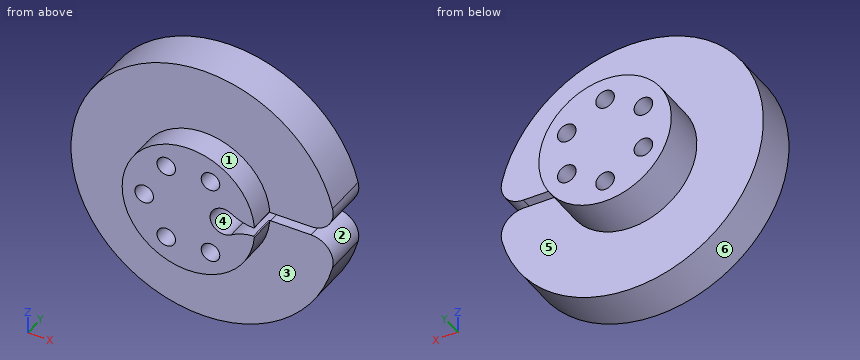
from build123d import *

# Parameters (mm, degrees)
SKETCH_1_R          = 30
EXTRUDE_1_DEPTH     = 10
SKETCH_2_R          = 14.975
EXTRUDE_2_DEPTH     = 10
EXTRUDE_START       = 6
SKETCH_3_R          = 14.975
EXTRUDE_3_DEPTH     = 6
SKETCH_4_R          = 2.1
CUT_EXTRUDE_1_DEPTH = 16
CUT_EXTRUDE_3_DEPTH = 46.343136195
FILLET_1_R          = 10
FILLET_2_R          = 5
FILLET_3_R          = 0.2
SKETCH_7_R          = 1.25
CUT_EXTRUDE_4_DEPTH = 8
SKETCH_8_R          = 2.1
CUT_EXTRUDE_5_DEPTH = 5


with BuildPart() as part:
    # 草图1 → 凸台-拉伸1 (new body)
    with BuildSketch(Plane(origin=(0, 0, 0), x_dir=(1, 0, 0), z_dir=(0, 1, 0))):
        with Locations(Location((0, 0, 0), (0, 0, 270))):
            Circle(SKETCH_1_R)
    extrude(amount=EXTRUDE_1_DEPTH)

    # 草图2 → 凸台-拉伸2 (add)
    with BuildSketch(Plane(origin=(0, 10, 0), x_dir=(1, 0, 0), z_dir=(0, 1, 0))):
        with Locations(Location((0, 0, 0), (0, 0, 270))):
            Circle(SKETCH_2_R)
    extrude(amount=EXTRUDE_2_DEPTH)

    # 草图3 → 凸台-拉伸3 (add)
    with BuildSketch(Plane.XZ.offset(EXTRUDE_START)):
        with Locations(Location((0, 0, 0), (0, 0, 90))):
            Circle(SKETCH_3_R)
    extrude(amount=-EXTRUDE_3_DEPTH)

    # 草图4 → 切除-拉伸1 (cut)
    with BuildSketch(Plane.XZ.offset(6)):
        with Locations(Location((-10, 0, 0), (0, 0, 270))):
            Circle(SKETCH_4_R)
        with Locations(Location((-5, 8.660254038, 0), (0, 0, 270))):
            Circle(SKETCH_4_R)
        with Locations(Location((5, 8.660254038, 0), (0, 0, 270))):
            Circle(SKETCH_4_R)
        with Locations(Location((5, -8.660254038, 0), (0, 0, 270))):
            Circle(SKETCH_4_R)
        with Locations(Location((-5, -8.660254038, 0), (0, 0, 270))):
            Circle(SKETCH_4_R)
    extrude(amount=-CUT_EXTRUDE_1_DEPTH, mode=Mode.SUBTRACT)

    # 草图6 → 切除-拉伸3 (cut, through all)
    with BuildSketch(Plane(origin=(0, 10, 0), x_dir=(1, 0, 0), z_dir=(0, 1, 0))):
        with BuildLine():
            Line((10.93428015, 1), (30.93428015, 1))
            Line((30.93428015, 1), (30.93428015, -1))
            Line((30.93428015, -1), (10.93428015, -1))
            ThreePointArc((10.93428015, -1), (4.9, 0), (10.93428015, 1))
        make_face()
    extrude(amount=-CUT_EXTRUDE_3_DEPTH, mode=Mode.SUBTRACT)

    # 圆角1
    # the kernel refuses this fillet: 10 mm, written as the material it takes off along each edge
    with BuildSketch(Plane(origin=(10.93428015, 10, -1), x_dir=(1, 0, 0), z_dir=(0, -1, 0))) as fillet_1_piece_1:
        with BuildLine():
            CenterArc((4.179790415, -10), FILLET_1_R, 90, 32.892109865)
            ThreePointArc((-1.250797803, -1.603053435), (-0.490230703, -0.906992999), (0, 0))
            Line((0, 0), (4.179790415, 0))
        make_face()
    extrude(amount=26.449476036, mode=Mode.SUBTRACT)
    with BuildSketch(Plane(origin=(10.93428015, 10, 1), x_dir=(1, 0, 0), z_dir=(0, -1, 0))) as fillet_1_piece_2:
        with BuildLine():
            CenterArc((4.179790415, 10), FILLET_1_R, 237.107890135, 32.892109865)
            ThreePointArc((-1.250797803, 1.603053435), (-0.490230703, 0.906992999), (0, 0))
            Line((0, 0), (4.179790415, 0))
        make_face()
    extrude(amount=26.449476036, mode=Mode.SUBTRACT)

    # 圆角2
    fillet_2_edges = [part.edges().sort_by_distance(p)[0] for p in [
        (29.983328701, 5, -1),
        (29.983328701, 5, 1),
    ]]
    fillet(fillet_2_edges, radius=FILLET_2_R)

    # 圆角3
    fillet_3_edges = [part.edges().sort_by_distance(p)[0] for p in [
        (14.941473943, -3, 1.001489591),
        (14.941473943, -3, -1.001489591),
    ]]
    fillet(fillet_3_edges, radius=FILLET_3_R)

    # 草图7 → 切除-拉伸4 (cut)
    with BuildSketch(Plane.XZ.offset(-10)):
        with Locations(Location((8, 0, 0), (0, 0, 270))):
            Circle(SKETCH_7_R)
    extrude(amount=-CUT_EXTRUDE_4_DEPTH, mode=Mode.SUBTRACT)

    # 草图8 → 切除-拉伸5 (cut)
    with BuildSketch(Plane(origin=(0, 20, 0), x_dir=(1, 0, 0), z_dir=(0, 1, 0))):
        with Locations(Location((-8.660254038, 5, 0), (0, 0, 270))):
            Circle(SKETCH_8_R)
        with Locations(Location((0, 10, 0), (0, 0, 270))):
            Circle(SKETCH_8_R)
        with Locations(Location((8.660254038, 5, 0), (0, 0, 270))):
            Circle(SKETCH_8_R)
        with Locations(Location((8.660254038, -5, 0), (0, 0, 270))):
            Circle(SKETCH_8_R)
        with Locations(Location((0, -10, 0), (0, 0, 270))):
            Circle(SKETCH_8_R)
        with Locations(Location((-8.660254038, -5, 0), (0, 0, 270))):
            Circle(SKETCH_8_R)
    extrude(amount=-CUT_EXTRUDE_5_DEPTH, mode=Mode.SUBTRACT)


solid = part.part
Verification items for the finished model (mm, model axes). Face numbers are marked on the shaded views. A direction names the side the tool comes from. Coordinates: 2 decimals unless noted, no trailing zeros. Write each loop counter-clockwise with the first axis right and the second up, starting at its lowest first coordinate (ties: lowest second). Pieces come first, ordered by that corner, then holes. Notation, with made-up numbers: (40, 5) - (80, 5) arc R16 cw to (80, 24) - close; hole circle Ø1 at (40, -16.75). An arc over 180 degrees is marked (long way). Answer as a JSON object with one key per item and string values.
(1) Tool access check on the marked faces 5 and 6. Record the directions out of +Z, -Z, +X, -X, +Y, -Y that give a thin tool (end or side, any length) a straight path to the whole face; none if there is none.
Report:
{"face 5": "+Y", "face 6": "+Y, -Y"}
(2) Thickness scan on line 1 along Z through (x, y) = (-4, 9); line 2 along X through (y, z) = (18, 5); line 3 along Y through (x, z) = (-11.5, -17). Record the ranges inside material, lowest first.
Report:
{"line 1": "-29.73 to -10.51, -6.81 to 6.81, 10.51 to 29.73", "line 2": "-14.12 to -10.76, -6.56 to 6.56, 10.76 to 14.12", "line 3": "0 to 10"}
(3) Mould release check, pull along X, two halves, no side actions. Record for the marked faces 1, 2, 3 and 4: pulls with the +X half, pulls with the -X half, needs draft (parallel to the pull), parting line crosses it, or undercut.
Report:
{"face 1": "parting line crosses it", "face 2": "pulls with the +X half", "face 3": "needs draft", "face 4": "undercut"}
(4) Cross-section at D-D on x = -10. Record the cut outline in (y, z), plus the area to 3 significant figures.
Report:
{"outline": "(-6, -11.15) - (0, -11.15) - (0, -28.28) - (10, -28.28) - (10, -11.15) - (20, -11.15) - (20, -6.62) - (15, -6.62) - (15, -3.38) - (20, -3.38) - (20, 3.38) - (15, 3.38) - (15, 6.62) - (20, 6.62) - (20, 11.15) - (10, 11.15) - (10, 28.28) - (0, 28.28) - (0, 11.15) - (-6, 11.15) - (-6, 2.1) - (10, 2.1) - (10, -2.1) - (-6, -2.1) - close", "area": "823 mm^2"}
(5) Cross-section at B-B on z = 5. Record the cut outline in (x, y).
Report:
{"outline": "(-29.58, 0) - (-14.12, 0) - (-14.12, -6) - (14.12, -6) - (14.12, 0) - (29.17, 0) - (29.17, 10) - (14.12, 10) - (14.12, 20) - (10.76, 20) - (10.76, 15) - (6.56, 15) - (6.56, 20) - (-6.56, 20) - (-6.56, 15) - (-10.76, 15) - (-10.76, 20) - (-14.12, 20) - (-14.12, 10) - (-29.58, 10) - close"}
(6) Gauge pin test, flat ends, axial feed: pin 1 Ø10 at (x, y) = (-2, 6.5) entering from -Z; pin 2 Ø12 at (y, z) = (5.5, 21.5) entering from -X; pin 3 Ø2 at (x, z) = (-0.5, 9.5) entering from +Y. Record the tip position at first contact, or that the pin passes through.
Report:
{"pin 1": "z = -30", "pin 2": "x = -25.69", "pin 3": "y = 15"}
(7) Cross-section at A-A on y = 3.5. Record the cut outline in (x, z), plus the area to 3 significant figures.
Report:
{"outline": "(9.68, -2.6) arc R3.1 cw (long way) to (9.68, 2.6) arc R10 ccw to (15.11, 1) - (24.27, 1) arc R5 ccw to (29.12, 7.2) arc R30 ccw (long way) to (29.12, -7.2) arc R5 ccw to (24.27, -1) - (15.11, -1) arc R10 ccw to start; hole circle Ø4.2 at (-10, 0); hole circle Ø4.2 at (-5, -8.66); hole circle Ø4.2 at (-5, 8.66); hole circle Ø4.2 at (5, -8.66); hole circle Ø4.2 at (5, 8.66)", "area": "2,670 mm^2"}
(8) Cross-section at C-C on y = 11.5. Record the cut outline in (x, z) (3 decimals), plus the area to 3 significant figures.
Report:
{"outline": "circle Ø29.95 at (0, 0); hole circle Ø2.5 at (8, 0)", "area": "700 mm^2"}
